Read the model definition and answer for the solid it produces. Units are mm, in the model's axes. Face numbers are marked on the shaded views. A direction names the side the tool comes from. Round coordinates to 2 decimals unless told otherwise and drop trailing zeros. Order: outer loops, then holes, each group sorted by start corner. A loop starts at its lowest first (then second) coordinate and runs counter-clockwise, first axis right, second up. Notation, with made-up numbers: (-28.75, 24.5) -> (-21.75, 24.5) arc R27 cw to (-21.75, 46.5) -> close; hole circle Ø5 at (-27.5, 63). An arc over 180 degrees is marked (long way). Use a Markdown table: item, result. Add a question column.
1. Consider L1, parallel to X at y = 29, z = 2.3; L2, parallel to Y at x = -48, z = 2.2; L3, parallel to X at y = 29.5, z = 0.95. Determine where each line is inside the solid, lowest interval first. Write a range as [from, to].
2. Given pin 1 (1.5 mm diameter, centred on y = 2.5, z = 4.5, fed in from -X); pin 2 (1.5 mm diameter, centred on x = -18.5, z = 4.5, fed in from -Y); pin 3 (1 mm diameter, centred on y = 34.5, z = 2.5, fed in from +X), each flat-ended and moving along its own axis, determine where each tip first touches the part or whether it passes through.
3. Section B-B, the plane x = -24.5 is taken. Give the number of separate pieces and of enclosed holes in the cut face, then the cut area to 3 significant figures.
4. For the marked faces 3 and 4, determine the directions among +Z, -Z, +X, -X, +Y, -Y from which every point of the face is accessible in a straight line to the end or side of a thin tool.
5. The mould has two halves that part along X. Classify the marked faces 1 and 2: +X half, -X half, draft (parallel to the pull), parting line (faces both ways), or undercut.
6. Section A-A, the plane z = 1.9 is taken. Give the vertices of the cut face in (x, y).
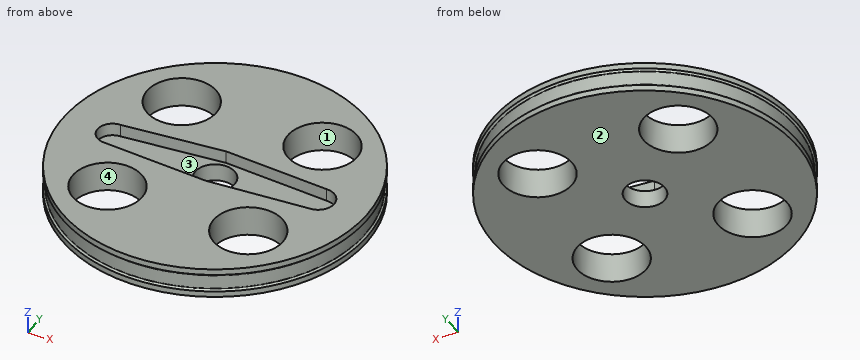
```python
from build123d import *

# Parameters (mm, degrees)
SKETCH1_R           = 25
BOSS_EXTRUDE1_DEPTH = 5
FILLET1_R           = 0.3
CUT_EXTRUDE1_DEPTH  = 2.1
SKETCH15_R          = 3.25
CUT_EXTRUDE2_DEPTH  = 10.1
SKETCH18_R          = 5.702447769
CUT_EXTRUDE4_DEPTH  = 10.1


with BuildPart() as part:
    # Sketch1 → Boss-Extrude1 (new body)
    with BuildSketch(Plane.XY):
        with Locations((-38.308088976, 20.909831899)):
            Circle(SKETCH1_R)
    extrude(amount=BOSS_EXTRUDE1_DEPTH)

    # Sketch12 → Cut-Revolve1 (revolve, cut)
    with BuildSketch(Plane.ZY.offset(38.308088976), mode=Mode.PRIVATE) as cut_revolve1_sk:
        Polygon((2.5, 45.909831899), (4, 45.909831899), (4, 45.609831899), (2.5, 45.609831899), (1, 45.609831899), (1, 45.909831899), align=None)
    revolve(cut_revolve1_sk.sketch.rotate(Axis((-38.308088976, 20.909831899, 0), (0, 0, 1)), 90), axis=Axis((-38.308088976, 20.909831899, 0), (0, 0, 1)), mode=Mode.SUBTRACT)

    # Fillet1
    fillet1_edges = [part.edges().sort_by_distance(p)[0] for p in [
        (-13.608088976, 20.909831899, 1),
        (-13.608088976, 20.909831899, 4),
    ]]
    fillet(fillet1_edges, radius=FILLET1_R - 0.0001)  # a hair under: the kernel refuses the full size

    # Sketch13 → Cut-Extrude1 (cut)
    with BuildSketch(Plane.XY.offset(5)):
        with BuildLine():
            Line((-38.537840804, 24.839400282), (-55.145400599, 23.363683745))
            ThreePointArc((-55.145400599, 23.363683745), (-57.599252444, 20.909831899), (-55.145400599, 18.455980054))
            Line((-55.145400599, 18.455980054), (-37.86715674, 17.168664797))
            Line((-37.86715674, 17.168664797), (-21.363574888, 18.259831899))
            ThreePointArc((-21.363574888, 18.259831899), (-18.713574888, 20.909831899), (-21.363574888, 23.559831899))
            Line((-21.363574888, 23.559831899), (-38.537840804, 24.839400282))
        make_face()
    extrude(amount=-CUT_EXTRUDE1_DEPTH, mode=Mode.SUBTRACT)

    # Sketch15 → Cut-Extrude2 (cut)
    with BuildSketch(Plane.XY.offset(2.9)):
        with Locations((-38.308088976, 20.909831899)):
            Circle(SKETCH15_R)
    extrude(amount=-CUT_EXTRUDE2_DEPTH, mode=Mode.SUBTRACT)

    # Sketch18 → Cut-Extrude4 (cut)
    with BuildSketch(Plane.XY.offset(5)):
        with Locations((-26.7425748, 32.475346075)):
            Circle(SKETCH18_R)
        with Locations((-26.7425748, 9.344317724)):
            Circle(SKETCH18_R)
        with Locations((-49.873603152, 9.344317724)):
            Circle(SKETCH18_R)
        with Locations((-49.873603152, 32.475346075)):
            Circle(SKETCH18_R)
    extrude(amount=-CUT_EXTRUDE4_DEPTH, mode=Mode.SUBTRACT)


solid = part.part
```
Verdict:
| question | item | result |
|---|---|---|
| 1 | L1 | x = [-61.65, -54.39], [-45.35, -31.26], [-22.22, -14.97] |
| 1 | L2 | y = [-1.81, 3.96], [14.73, 27.09], [37.86, 43.63] |
| 1 | L3 | x = [-61.79, -54.74], [-45.01, -31.61], [-21.88, -14.83] |
| 2 | pin 1 | stops at x = -56 |
| 2 | pin 2 | stops at y = 4.73 |
| 2 | pin 3 | stops at x = -17.36 |
| 3 | separate pieces | 3 |
| 3 | enclosed holes | 0 |
| 3 | area | 89.4 mm2 |
| 4 | face 3 | +Z |
| 4 | face 4 | +Z, -Z |
| 5 | face 1 | undercut |
| 5 | face 2 | draft |
| 6 | outline | circle Ø49.4 at (-38.31, 20.91); hole circle Ø11.4 at (-49.87, 9.34); hole circle Ø11.4 at (-49.87, 32.48); hole circle Ø6.5 at (-38.31, 20.91); hole circle Ø11.4 at (-26.74, 9.34); hole circle Ø11.4 at (-26.74, 32.48) |
